Could you check a few things on this model? Use its own coordinates, in mm. Coordinates: 2 decimals unless noted, no trailing zeros. Write each loop counter-clockwise with the first axis right and the second up, starting at its lowest first coordinate (ties: lowest second). Pieces come first, ordered by that corner, then holes. Notation, with made-up numbers: M 60.25,8 L 76.25,8 A18 ccw 76.25,23 Z; hole C -31.75,22 d3. An arc over 180 degrees is marked long. Answer as CSV lines item,"result". Start each with the question number.
Item 1: Suppose I cut it at B-B, the plane x = 15. Write out the boundary of the cut face in (y, z).
Item 2: I'm going to push flat-ended pins straight in: P1, Ø1, axis at x = 43, y = 61, coming from the +Z side; P2, Ø3, axis at x = 77.5, z = 1126.5, coming from the -Y side; P3, Ø10, axis at x = 78.5, y = 69.5, coming from the +Z side. Where does each tip first touch, or does it pass through?
Item 3: If I drill on line 1 along Y through (x, z) = (78.74, 1634); line 2 along X through (y, z) = (67, 1303); line 3 along X through (y, z) = (67, 1640), over which ranges is the centre line in solid material (lowest first)? Write a range as [from, to].
Item 4: Suppose I cut it at A-A, the plane z = 1089. Write out the boundary of the cut face in (x, y).
```python
from build123d import *

# Parameters (mm, degrees)
SKETCH1_W           = 157.48
SKETCH1_H           = 134.62
BOSS_EXTRUDE1_DEPTH = 586.74
SKETCH2_R           = 25.4
SKETCH2_R_2         = 6.35
BOSS_EXTRUDE2_DEPTH = 1016
SKETCH3_R           = 31.75
SKETCH3_R_2         = 25.4
BOSS_EXTRUDE3_DEPTH = 76.2


with BuildPart() as part:
    # Sketch1 → Boss-Extrude1 (new body)
    with BuildSketch(Plane.XY):
        with Locations((78.74, 67.31)):
            Rectangle(SKETCH1_W, SKETCH1_H)
    extrude(amount=BOSS_EXTRUDE1_DEPTH)

    # Sketch2 → Boss-Extrude2 (add)
    with BuildSketch(Plane.XY.offset(586.74)):
        with Locations((78.74, 67.31)):
            Circle(SKETCH2_R)
        with Locations((78.74, 67.31)):
            Circle(SKETCH2_R_2, mode=Mode.SUBTRACT)
    extrude(amount=BOSS_EXTRUDE2_DEPTH)

    # Sketch3 → Boss-Extrude3 (add, symmetric)
    with BuildSketch(Plane.XY.offset(1602.74)):
        with Locations(Location((78.74, 67.31, 0), (0, 0, 180))):
            Circle(SKETCH3_R)
        with Locations((78.74, 67.31)):
            Circle(SKETCH3_R_2, mode=Mode.SUBTRACT)
    extrude(amount=BOSS_EXTRUDE3_DEPTH, both=True)


solid = part.part
```
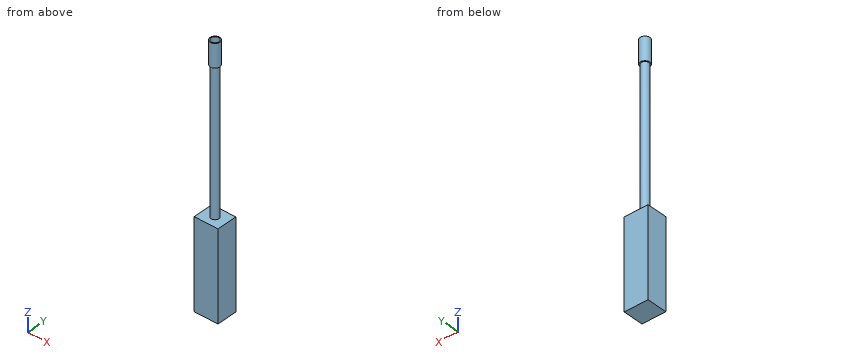
Ans:
1,outline,"M 0,0 L 134.62,0 L 134.62,586.74 L 0,586.74 Z"
2,P1,"stops at z = 586.74"
2,P2,"stops at y = 41.91"
2,P3,"stops at z = 1602.74"
3,line 1,"y = [35.56, 41.91], [92.71, 99.06]"
3,line 2,"x = [53.34, 72.4], [85.08, 104.14]"
3,line 3,"x = [46.99, 53.34], [104.14, 110.49]"
4,outline,"C 78.74,67.31 d50.8; hole C 78.74,67.31 d12.7"
